Autodesk Inventor part; units mm, degrees
ref_plane "YZ Plane" through (0, 0, 0) normal (1, 0, 0) x (0, 1, 0)
ref_plane "XZ Plane" through (0, 0, 0) normal (0, 1, 0) x (-1, 0, 0)
ref_plane "XY Plane" through (0, 0, 0) normal (0, 0, 1) x (1, 0, 0)
sketch "Sketch1" plane through (0, 0, 0) normal (0, 1, 0) x (-1, 0, 0)
  line L0 (0, 0) -> (-50, 0)
  line L1 (-50, 0) -> (-50, -105)
  line L2 (-50, -105) -> (0, -105)
  line L3 (0, -105) -> (0, 0)
  line L4 (2, 2) -> (-52, 2)
  line L5 (-52, 2) -> (-52, -104)
  line L6 (2, -104) -> (2, 2)
  line L7 (2, -104) -> (2, -111)
  line L8 (2, -111) -> (-52, -111)
  line L9 (-52, -111) -> (-52, -102)
  dimension "d0" = 50
  dimension "d1" = 105
  dimension "d23" = 6
  dimension "d24" = 2
extrude "Extrusion1" add sketch "Sketch1" along normal blind 2
ref_plane "Work Plane1" through (45, 2, -25) normal (0, 0.9999, -0.0117) x (-1, 0, 0)
sketch "Sketch3" plane through (45, 2, -25) normal (0, 0.9999, -0.0117) x (-1, 0, 0)
  line L0 (51, 33) -> (-14, 33)
  line L1 (-14, 33) -> (-14, -92)
  line L2 (-14, -92) -> (51, -92)
  line L3 (51, -92) -> (51, 33)
  point P0 (45, 24.9749)
extrude "Extrusion3" cut sketch "Sketch3" along normal blind 2
sketch "Sketch7" plane through (45, 2, -25) normal (0, 0.9999, -0.0117) x (-1, 0, 0)
  line L0 (47, -86.0175) -> (47, 26.9748)
  line L1 (47, -82) -> (-7, -82)
  line L2 (-7, -82) -> (-7, -84)
  line L3 (-7, -84) -> (47, -84)
  line L4 (47, -84) -> (47, -82)
  point P0 (45, 24.9749)
extrude "Extrusion6" cut sketch "Sketch7" against normal blind 0.5
sketch "Sketch8" plane through (0, 0, 0) normal (0, -1, 0) x (1, 0, 0)
  line L0 (50, -25) -> (50, 0) construction
  line L1 (50, 0) -> (50, -105) construction
  line L2 (50, -105) -> (50, -25) construction
  line L3 (50, -25) -> (50, -105)
  line L4 (50, -25) -> (0, -25)
  line L5 (0, -25) -> (0, -23)
  line L6 (0, -23) -> (50, -23)
  line L7 (50, -23) -> (50, -25)
  point P0 (0, 0)
extrude "Extrusion7" add sketch "Sketch8" against normal blind 2
properties part number "wing1.1"
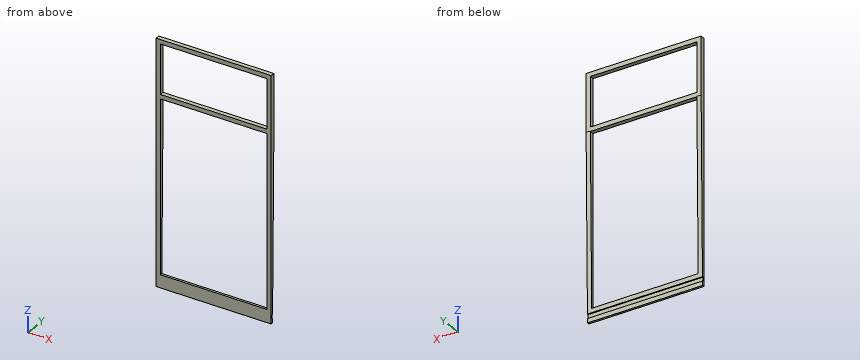
Source: CAD feature listing. Evaluate the final solid. Frame: model axes, mm. Coordinates: 2 decimals unless noted, no trailing zeros. Loops run counter-clockwise (first coordinate to the right, second up) from the corner with the lowest first, then second, coordinate; pieces in that order, holes last. Notation, with made-up numbers: (21, 71) - (78, 71) arc R34 ccw to (78, 104) - close; hole circle Ø3 at (58.25, 84). An arc over 180 degrees is marked (long way). Return JSON: item names as keys, results as strings.
Q1. Section C-C, the plane y = 1.45. Return loops of the section in (x, z).
Results:
{"outline": "(-2, -71.83) - (0, -71.83) - (0, -25) - (50, -25) - (50, -71.83) - (52, -71.83) - (52, 2) - (-2, 2) - close; hole (0, -23) - (50, -23) - (50, 0) - (0, 0) - close"}
Q2. Section B-B, the plane z = -11. Return loops of the section in (x, y), plus the area to 3 significant figures.
Results:
{"outline": "(-2, 0) - (0, 0) - (0, 2) - (-2, 2) - close; (50, 0) - (52, 0) - (52, 2) - (50, 2) - close", "area": "8.00 mm2"}
Q3. Material intervals for line 1 along Z through (x, y) = (49.5, 0.2); line 2 along Z through (x, y) = (44, 0.85); line 3 along Z through (x, y) = (48, 1.8), sorted ascending.
Results:
{"line 1": "-111 to -105, -25 to -23, 0 to 2", "line 2": "-111 to -108.99, -106.99 to -105, -25 to -23, 0 to 2", "line 3": "-25 to -23, 0 to 2"}
Q4. Section A-A, the plane x = 42.5. Return loops of the section in (y, z).
Results:
{"outline": "(0, -111) - (0.99, -111) - (1.02, -108.99) - (0.52, -108.99) - (0.54, -106.99) - (1.04, -106.99) - (1.06, -105) - (0, -105) - close; (0, -25) - (2, -25) - (2, -23) - (0, -23) - close; (0, 0) - (2, 0) - (2, 2) - (0, 2) - close"}
Q5. Section D-D, the plane z = -76. Return loops of the section in (x, y), plus the area to 3 significant figures.
Results:
{"outline": "(-2, 0) - (0, 0) - (0, 1.4) - (-2, 1.4) - close; (50, 0) - (52, 0) - (52, 1.4) - (50, 1.4) - close", "area": "5.60 mm2"}
